Geometry: final body of the model. Coordinates: model frame, mm. A direction names the side the tool comes from. Give positions to 0.01 mm unless a question says otherwise; leave off trailing zeros. Order: outer loops, then holes, each group sorted by start corner. A loop starts at its lowest first (then second) coordinate and runs counter-clockwise, first axis right, second up. Notation, with made-up numbers: (3, 1.25) -> (22, 1.25) arc R27 cw to (22, 38.25) -> close; hole circle Ø9 at (-2.5, -3.5). An arc over 180 degrees is marked (long way). Write item = value, one per line.
Solid Edge part; units mm, degrees
sketch "Sketch1" plane through (0, 0, 0) normal (0, -1, 0) x (1, 0, 0)
  line L0 (-8.64, -6.23) -> (8.64, -6.23)
  line L1 (8.64, 4.23) -> (8.64, -6.23)
  line L2 (8.64, 4.23) -> (10.455, 4.23)
  line L3 (10.455, 4.23) -> (10.455, 6.23)
  line L4 (10.455, 6.23) -> (-10.455, 6.23)
  line L5 (-10.455, 6.23) -> (-10.455, 4.23)
  line L6 (-10.455, 4.23) -> (-8.64, 4.23)
  line L7 (-8.64, 4.23) -> (-8.64, -6.23)
extrude "Protrusion1" add sketch "Sketch1" along normal mid plane 15
sketch "Sketch2" plane through (0, 0, -6.23) normal (0, 0, -1) x (0, 1, 0)
  line L0 (-6.17, -8.64) -> (-7.5, -8.64)
  line L1 (-7.5, -8.64) -> (-7.5, 8.64)
  line L2 (-7.5, 8.64) -> (-6.17, 8.64)
  line L3 (-6.17, -8.64) -> (-6.17, 8.64)
  line L4 (6.17, 8.64) -> (7.5, 8.64)
  line L5 (7.5, 8.64) -> (7.5, -8.64)
  line L6 (7.5, -8.64) -> (6.17, -8.64)
  line L7 (6.17, 8.64) -> (6.17, -8.64)
extrude "Cutout1" cut sketch "Sketch2" against normal up to surface (10.46 mm away)
sketch "Sketch3" plane through (0, 0, -6.23) normal (0, 0, -1) x (1, 0, 0)
  line L0 (-7.44, -5) -> (-6.64, -5)
  line L1 (-6.64, -5) -> (-6.64, 5)
  line L2 (-6.64, 5) -> (-7.44, 5)
  line L3 (-7.44, 5) -> (-7.44, -5)
  line L4 (-0.44, -5) -> (0.36, -5)
  line L5 (0.36, -5) -> (0.36, 5)
  line L6 (0.36, 5) -> (-0.44, 5)
  line L7 (-0.44, 5) -> (-0.44, -5)
  dimension "D1" = 6.64
extrude "ExtrudedProtrusion_2" add sketch "Sketch3" along normal blind 7.2684 and the other way blind 4.6435
sketch "Sketch4" plane through (0, 0, 0) normal (0, -1, 0) x (1, 0, 0)
  spline S0 degree 3 poles (-7.0557, 6.23) (-7.8479, 7.243) (-7.9337, 8.5637) (-7.3131, 10.1922) knots 0 0 0 0 1 1 1 1
  spline S1 degree 3 poles (-7.3131, 10.1922) (-6.0411, 9.5159) (-2.945, 7.8753) (2.3147, 6.9676) (5.6977, 6.5935) (7.05, 6.4683) knots 0 0 0 0 0.262711 0.752323 1 1 1 1
  line L0 (7.05, 6.4683) -> (7.05, 6.23)
  line L1 (7.05, 6.23) -> (-7.037, 6.23)
  line L2 (-7.0557, 6.23) -> (-7.037, 6.23)
extrude "ExtrudedProtrusion_3" add sketch "Sketch4" along normal mid plane 12
fillet "Round_1" radius 0.5 1 edges at (-7.3131, 0, 10.1922)
1) Line query: line 1 (Z direction, x = 5, y = 7); line 2 (Y direction, x = 4.75, z = 2); line 3 (X direction, y = -1.75, z = -7.75). Output: solid intervals per line, ascending. Write a range as from..to.
Check sheet entries:
line_1 = 4.23..6.23
line_2 = -6.17..6.17
line_3 = -7.44..-6.64, -0.44..0.36
2) Mould query, pull axis X, two halves, no side actions, for faces 5 (the face through (-8.64, 0, -1)), 6 (the face through (0, -7.5, 5)), 7 (the face through (-6.64, 0, -10)). Classes: +X half, -X half, draft (parallel to the pull), parting line (faces both ways), or undercut.
Check sheet entries:
face_5 = -X half
face_6 = draft
face_7 = undercut
3) Section query B-B (z = -3). Output: boundary loops of the cut face in (x, y).
Check sheet entries:
outline = (-8.64, -6.17) -> (8.64, -6.17) -> (8.64, 6.17) -> (-8.64, 6.17) -> close
4) First-contact query: P1, Ø5, axis at y = -4.5, z = -9.5, coming from the -X side; P2, Ø3, axis at x = -4.5, y = -2.5, coming from the -Z side; P3, Ø3, axis at x = -2, z = 8.5, coming from the -Y side. Flat tips, straight axial feed; report the tip coordinate or a pass-through.
Check sheet entries:
P1 = -7.44
P2 = -6.23
P3 = -6
5) Section query A-A (z = -9). Output: boundary loops of the cut face in (x, y).
Check sheet entries:
outline = (-7.44, -5) -> (-6.64, -5) -> (-6.64, 5) -> (-7.44, 5) -> close; (-0.44, -5) -> (0.36, -5) -> (0.36, 5) -> (-0.44, 5) -> close
6) Reachability of faces 1 (the face through (0.36, 0, -10)), 2 (the face through (-7.44, 0, -10)), 3 (the face through (0, 5, -10)), 4 (the face through (0, -6.17, -1)) from +Z, -Z, +X, -X, +Y, -Y: full face, straight path, thin tool, end or side. Return the list, or none.
Check sheet entries:
face_1 = -Z, +X, +Y, -Y
face_2 = -Z, -X, +Y, -Y
face_3 = -Z, +X, -X, +Y
face_4 = -Z, +X, -X, -Y
